Can you work these out from the model? Positions are in its coordinate system, mm. Give positions to 0.01 mm unless a question says otherwise; leave off trailing zeros. Loops run counter-clockwise (first coordinate to the right, second up) from the corner with the lowest first, then second, coordinate; pieces in that order, holes last.
from build123d import *

# Parameters (mm, degrees)
SKETCH1_R           = 14.8209
BOSS_EXTRUDE1_DEPTH = 42.6212
HOLE1_D             = 19.05
HOLE4_D             = 9.525
CHAMFER1_SIZE       = 1.524


with BuildPart() as part:
    # Sketch1 → Boss-Extrude1 (new body)
    with BuildSketch(Plane(origin=(0, 0, 0), x_dir=(0, 0, -1), z_dir=(1, 0, 0))):
        Circle(SKETCH1_R)
    extrude(amount=BOSS_EXTRUDE1_DEPTH)

    # Hole1 (through all)
    with Locations(Plane(origin=(42.6212, 0, 0), x_dir=(0, 0, -1), z_dir=(1, 0, 0))):
        with Locations((0, 0)):
            Hole(HOLE1_D / 2)

    # Hole4 (through all)
    with Locations(Plane(origin=(12.7, 0, 14.8209), x_dir=(1, 0, 0), z_dir=(0, 0, 1))):
        with Locations((0, 0)):
            Hole(HOLE4_D / 2)

    # Chamfer1
    chamfer1_edges = [part.edges().sort_by_distance(p)[0] for p in [
        (0, 0, 14.8209),
    ]]
    chamfer(chamfer1_edges, length=CHAMFER1_SIZE)


solid = part.part
(1) Please list where these lines run through material, in increasing order: probe 1 along Z at (x, y) = (30, 0) (3 decimals); probe 2 along X at (y, z) = (0, -13.25).
Returned:
probe 1: z = -14.821 to -9.525, 9.525 to 14.821
probe 2: x = 0 to 7.94, 17.46 to 42.62
(2) Will these pins go through, and if not, where does the flat tip stop? P1, Ø6, axis at x = 5.5, y = -10.5, coming from the +Z side; P2, Ø17, axis at y = 0, z = 0, coming from the +X side; P3, Ø8, axis at x = 12.5, y = -11, coming from the +Z side; P4, Ø6, axis at x = 37.5, y = 7, coming from the -Z side.
Returned:
P1: stops at z = 12.78
P2: passes through
P3: stops at z = 13.06
P4: stops at z = -14.27
(3) Suppose I cut it at D-D on x = 19. List the corners of the cut face in (y, z) for me (3 decimals), plus the area to 3 significant figures.
Returned:
outline: circle Ø29.642 at (0, 0); hole circle Ø19.05 at (0, 0)
area: 405 mm2
(4) Suppose I cut it at A-A on z = 0. List the corners of the cut face in (x, y) for me (3 decimals), plus the area to 3 significant figures.
Returned:
outline: (0, -13.297) - (1.524, -14.821) - (42.621, -14.821) - (42.621, -9.525) - (0, -9.525) - close; (0, 9.525) - (42.621, 9.525) - (42.621, 14.821) - (1.524, 14.821) - (0, 13.297) - close
area: 449 mm2
(5) Thinking about a two-plate mould opening in X: for faces 1 (the flat face through (42.621, -10, 0)), 2 (the flat face through (0, -9, -6)), 3 (the cylindrical face through (16.48, -2.9, 11.49)), which applies, pulls with the +X half, pulls with the -X half, needs draft (parallel to the pull), parting line crosses it, or undercut?
Returned:
face 1: pulls with the +X half
face 2: pulls with the -X half
face 3: undercut
(6) Suppose I cut it at B-B on y = 0. List the corners of the cut face in (x, z) for me (1 decimal).
Returned:
outline: (0, -13.3) - (1.5, -14.8) - (7.9, -14.8) - (7.9, -9.5) - (0, -9.5) - close; (0, 9.5) - (7.9, 9.5) - (7.9, 14.8) - (1.5, 14.8) - (0, 13.3) - close; (17.5, -14.8) - (42.6, -14.8) - (42.6, -9.5) - (17.5, -9.5) - close; (17.5, 9.5) - (42.6, 9.5) - (42.6, 14.8) - (17.5, 14.8) - close
